Could you check a few things on this model? Use its own coordinates, in mm. A direction names the side the tool comes from. Give positions to 0.01 mm unless a question says otherwise; leave off trailing zeros. Order: outer loops, then holes, each group sorted by start corner. A loop starts at its lowest first (then second) coordinate and runs counter-clockwise, first axis right, second up.
from build123d import *

# Parameters (mm, degrees)
F0_W     = 91.270662
F0_H     = 62.30978
F1_DEPTH = 50
F3_DEPTH = 55


with BuildPart() as f1:
    # F0 (on Front) → F1 (new body)
    with BuildSketch(Plane.XZ):
        Rectangle(F0_W, F0_H)
    extrude(amount=-F1_DEPTH)

    # F2 (on face) → F3 (cut)
    with BuildSketch(Plane.YZ.offset(45.635331)):
        Polygon((0, 31.15489), (0, -8.84511), (26.905989, -8.84511), (50, 31.15489), align=None)
    extrude(amount=-F3_DEPTH, mode=Mode.SUBTRACT)


solid = f1.part
Item 1: For pin 1 (8 mm diameter, centred on x = 23, y = 21.5, fed in from +Z), with a flat end and sliding along its axis, tell me the tip position at first contact or that it passes through.
Findings:
pin 1: stops at z = -8.85
Item 2: Imagine slicing it at B-B on x = 29. List the corners of the cut face in (y, z) for me.
Findings:
outline: (0, -31.15) - (50, -31.15) - (50, 31.15) - (26.91, -8.85) - (0, -8.85) - close
Item 3: Imagine slicing it at C-C on z = -3. List the corners of the cut face in (x, y) for me, then the cut area to 3 significant figures.
Findings:
outline: (-45.64, 0) - (-9.36, 0) - (-9.36, 30.28) - (45.64, 30.28) - (45.64, 50) - (-45.64, 50) - close
area: 2,900 mm2
Item 4: Please list where these lines run through material, in increasing order: line 1 along X through (y, z) = (23, 6.5); line 2 along Z through (x, y) = (10, 21); line 3 along Z through (x, y) = (23, 27).
Findings:
line 1: x = -45.64 to -9.36
line 2: z = -31.15 to -8.85
line 3: z = -31.15 to -8.68
Item 5: For faces 1 (the flat face through (45.635, 30, -14)), 2 (the flat face through (19, 13, -8.845)), which set-ups out of +Z, -Z, +X, -X, +Y, -Y let a thin tool reach every point of the face, with its end or its side?
Findings:
face 1: +Z, -Z, +X, +Y, -Y
face 2: +Z, +X, -Y
Item 6: Imagine slicing it at A-A on y = 23.5. List the corners of the cut face in (x, z) for me.
Findings:
outline: (-45.64, -31.15) - (45.64, -31.15) - (45.64, -8.85) - (-9.36, -8.85) - (-9.36, 31.15) - (-45.64, 31.15) - close
